from build123d import *

# Parameters (mm, degrees)
BASIS_LINEAR_AUSTRAGEN_DEPTH    = 19
AUFSATZ_LINEAR_AUSTRAGEN1_DEPTH = 14
AUFSATZ_LINEAR_AUSTRAGEN2_DEPTH = 14
SKIZZE4_R                       = 9.5
SCHNITT_LINEAR_AUSTRAGEN1_DEPTH = 57.056519098


with BuildPart() as part:
    # Skizze1 → Basis-Linear austragen (new body)
    with BuildSketch(Plane.XY):
        Polygon((11.547005384, -20), (23.094010768, 0), (11.547005384, 20), (-11.547005384, 20), (-23.094010768, 0), (-11.547005384, -20), align=None)
    extrude(amount=BASIS_LINEAR_AUSTRAGEN_DEPTH)

    # Skizze2 → Aufsatz-Linear austragen1 (add)
    with BuildSketch(Plane.XY.offset(19)):
        Polygon((7.505553499, -13), (15.011106999, 0), (7.505553499, 13), (-7.505553499, 13), (-15.011106999, 0), (-7.505553499, -13), align=None)
    extrude(amount=AUFSATZ_LINEAR_AUSTRAGEN1_DEPTH)

    # Skizze3 → Aufsatz-Linear austragen2 (add)
    with BuildSketch(Plane(origin=(0, 0, 0), x_dir=(-1, 0, 0), z_dir=(0, 0, -1))):
        Polygon((7.505553499, -13), (15.011106999, 0), (7.505553499, 13), (-7.505553499, 13), (-15.011106999, 0), (-7.505553499, -13), align=None)
    extrude(amount=AUFSATZ_LINEAR_AUSTRAGEN2_DEPTH)

    # Skizze4 → Schnitt-Linear austragen1 (cut, through all)
    with BuildSketch(Plane.XY.offset(33)):
        Circle(SKIZZE4_R)
    extrude(amount=-SCHNITT_LINEAR_AUSTRAGEN1_DEPTH, mode=Mode.SUBTRACT)


solid = part.part
Can you work these out from the model? Positions are in its coordinate system, mm. A direction names the side the tool comes from. Give positions to 0.01 mm unless a question says otherwise; leave off trailing zeros. Write each loop counter-clockwise with the first axis right and the second up, starting at its lowest first coordinate (ties: lowest second). Pieces come first, ordered by that corner, then holes. Notation, with made-up numbers: M 66.5,24 L 77.5,24 A23 cw 77.5,62 Z; hole C -25.5,-20 d8. An arc over 180 degrees is marked long. Answer in a Markdown table with one row per item. Add a question column.
Item 1: Imagine slicing it at B-B, the plane z = 12.5. Write out the boundary of the cut face in (x, y).
Item 2: Imagine slicing it at A-A, the plane x = 0. Write out the boundary of the cut face in (y, z).
Item 3: For pin 1 Ø12 at (x, y) = (-2, -15.5) entering from +Z; pin 2 Ø6 at (x, z) = (4, 27) entering from +Y; pin 3 Ø4 at (x, z) = (-2.5, -10.5) entering from -Y; pin 4 Ø6 at (x, y) = (16.5, -11) entering from +Z, each with a flat end and sliding along its axis, tell me the tip position at first contact or that it passes through.
Item 4: Imagine slicing it at D-D, the plane z = -1. Write out the boundary of the cut face in (x, y).
Item 5: We'd pull the mould along X, two halves only. Please class faces 1 (the flat face through (0, -20, 9)), 2 (the flat face through (17.24, -10.14, 9.37)), 3 (the cylindrical face through (4.38, -8.43, 9.83)): released by +X, released by -X, zero draft, split by the parting line, or undercut.
Item 6: Imagine slicing it at C-C, the plane y = 5.5. Write out the boundary of the cut face in (x, z).
Item 7: On a 3-axis mill with a long thin cutter (end or side, diameter ignored), from which of +Z, -Z, +X, -X, +Y, -Y can I reach the whole of each face in a straight line? I mean faces 4 (the flat face through (11.31, 6.41, 25.9)), 5 (the flat face through (10, 9, 19)), 6 (the flat face through (0, 13, -7)), 7 (the flat face through (0, 13, 26)), 8 (the flat face through (-11.2, 6.6, 25.9)). Say none if no direction works.
Item 8: Please list where these lines run through material, in increasing order: L1, parallel to Y at x = 0, z = -3; L2, parallel to Z at x = 2, y = 16; L3, parallel to Y at x = 4, z = 7.
Evaluation:
| question | item | result |
|---|---|---|
| 1 | outline | M -23.09,0 L -11.55,-20 L 11.55,-20 L 23.09,0 L 11.55,20 L -11.55,20 Z; hole C 0,0 d19 |
| 2 | outline | M -20,0 L -13,0 L -13,-14 L -9.5,-14 L -9.5,33 L -13,33 L -13,19 L -20,19 Z; M 9.5,-14 L 13,-14 L 13,0 L 20,0 L 20,19 L 13,19 L 13,33 L 9.5,33 Z |
| 3 | pin 1 | stops at z = 33 |
| 3 | pin 2 | stops at y = 13 |
| 3 | pin 3 | stops at y = -13 |
| 3 | pin 4 | stops at z = 19 |
| 4 | outline | M -15.01,0 L -7.51,-13 L 7.51,-13 L 15.01,0 L 7.51,13 L -7.51,13 Z; hole C 0,0 d19 |
| 5 | face 1 | zero draft |
| 5 | face 2 | released by +X |
| 5 | face 3 | undercut |
| 6 | outline | M -19.92,0 L -11.84,0 L -11.84,-14 L -7.75,-14 L -7.75,33 L -11.84,33 L -11.84,19 L -19.92,19 Z; M 7.75,-14 L 11.84,-14 L 11.84,0 L 19.92,0 L 19.92,19 L 11.84,19 L 11.84,33 L 7.75,33 Z |
| 7 | face 4 | +Z, +X, +Y |
| 7 | face 5 | +Z |
| 7 | face 6 | -Z, +X, -X, +Y |
| 7 | face 7 | +Z, +X, -X, +Y |
| 7 | face 8 | +Z, -X, +Y |
| 8 | L1 | y = -13 to -9.5, 9.5 to 13 |
| 8 | L2 | z = 0 to 19 |
| 8 | L3 | y = -20 to -8.62, 8.62 to 20 |
